from build123d import *

# Parameters (mm, degrees)
F0_W     = 57.15
F0_H     = 44.45
F1_DEPTH = 25.4
F2_R     = 12.7
F3_DEPTH = 25.4
F5_DEPTH = 12.7


with BuildPart() as f1:
    # F0 (on Front) → F1 (new body)
    with BuildSketch(Plane.XZ):
        with Locations((28.575, 22.225)):
            Rectangle(F0_W, F0_H)
    extrude(amount=-F1_DEPTH)

    # F2 (on face) → F3 (cut)
    with BuildSketch(Plane.XZ):
        with Locations((25.4, 22.225)):
            Circle(F2_R)
    extrude(amount=-F3_DEPTH, mode=Mode.SUBTRACT)

    # F4 (on face) → F5 (cut)
    with BuildSketch(Plane.XZ):
        with BuildLine():
            Line((24.5106721265, 34.8938237786), (35.8631740273, 15.0269454522))
            ThreePointArc((35.8631740273, 15.0269454522), (37.5279081079, 18.4562011295), (38.1, 22.225))
            ThreePointArc((38.1, 22.225), (34.0601251725, 31.5143612265), (24.5106721265, 34.8938237786))
        make_face()
        with BuildLine():
            Line((44.45, 0), (57.15, 0))
            Line((57.15, 0), (57.15, 44.45))
            Line((57.15, 44.45), (19.05, 44.45))
            Line((19.05, 44.45), (24.5106721265, 34.8938237786))
            ThreePointArc((24.5106721265, 34.8938237786), (34.0601251725, 31.5143612265), (38.1, 22.225))
            ThreePointArc((38.1, 22.225), (37.5279081079, 18.4562011295), (35.8631740273, 15.0269454522))
            Line((35.8631740273, 15.0269454522), (44.45, 0))
        make_face()
    extrude(amount=-F5_DEPTH, mode=Mode.SUBTRACT)


solid = f1.part
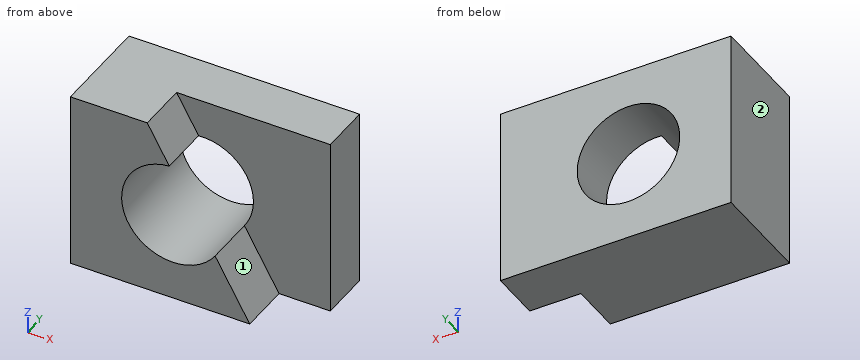
Here's how the part is built. I have some questions about the finished solid (model axes, mm). Face numbers are marked on the shaded views. A direction names the side the tool comes from. Coordinates: 2 decimals unless noted, no trailing zeros. Order: outer loops, then holes, each group sorted by start corner. A loop starts at its lowest first (then second) coordinate and runs counter-clockwise, first axis right, second up.
Item 1: If we section it at C-C on y = 3.5: List the corners of the cut face in (x, z) for me (3 decimals).
Result sheet:
outline: (0, 0) - (44.45, 0) - (35.863, 15.027) arc R12.7 cw (long way) to (24.511, 34.894) - (19.05, 44.45) - (0, 44.45) - close
Item 2: For the marked faces 1 and 2, which set-ups out of +Z, -Z, +X, -X, +Y, -Y let a thin tool reach every point of the face, with its end or its side?
Result sheet:
face 1: +Z, +X, -Y
face 2: +Z, -Z, -X, +Y, -Y
Item 3: If we section it at B-B on z = 21.5: List the corners of the cut face in (x, y) for me, plus the area to 3 significant figures.
Result sheet:
outline: (0, 0) - (12.72, 0) - (12.72, 25.4) - (0, 25.4) - close; (38.08, 12.7) - (57.15, 12.7) - (57.15, 25.4) - (38.08, 25.4) - close
area: 565 mm2
Item 4: I need wall thicknesses on line 1 (Z direction, x = 25.4, y = 17.75) (3 decimals); line 2 (Y direction, x = 49, z = 37); line 3 (X direction, y = 17, z = 22). Which ranges of each line are inside material? Lowest first, please.
Result sheet:
line 1: z = 0 to 9.525, 34.925 to 44.45
line 2: y = 12.7 to 25.4
line 3: x = 0 to 12.7, 38.1 to 57.15
Item 5: If we section it at D-D on x = 42.5: List the corners of the cut face in (y, z) for me, plus the area to 3 significant figures.
Result sheet:
outline: (0, 0) - (25.4, 0) - (25.4, 44.45) - (12.7, 44.45) - (12.7, 3.41) - (0, 3.41) - close
area: 608 mm2
Item 6: For P1, Ø5, axis at x = 50.5, z = 26.5, coming from the -Y side; P2, Ø10, axis at x = 23.5, z = 16.5, coming from the +Y side, each with a flat end and sliding along its axis, tell me the tip position at first contact or that it passes through.
Result sheet:
P1: stops at y = 12.7
P2: passes through
Item 7: If we section it at A-A on x = 25.4: List the corners of the cut face in (y, z) for me (3 decimals), plus the area to 3 significant figures.
Result sheet:
outline: (0, 0) - (25.4, 0) - (25.4, 9.525) - (0, 9.525) - close; (12.7, 34.925) - (25.4, 34.925) - (25.4, 44.45) - (12.7, 44.45) - close
area: 363 mm2
